from build123d import *

# Parameters (mm, degrees)
SKETCH1_R           = 2.45
SKETCH1_W           = 10
SKETCH1_H           = 3.175
SKETCH1_W_2         = 12
SKETCH1_H_2         = 2
BOSS_EXTRUDE1_DEPTH = 3.175


with BuildPart() as part:
    # Sketch1 → Boss-Extrude1 (new body)
    with BuildSketch(Plane(origin=(0, 0, 0), x_dir=(1, 0, 0), z_dir=(0, 1, 0))):
        Polygon((0, 0), (100, 0), (100, 10), (103.175, 10), (103.175, 20), (100, 20), (100, 80), (103.175, 80), (103.175, 90), (100, 90), (100, 100), (0, 100), (0, 90), (-3.175, 90), (-3.175, 80), (0, 80), (0, 20), (-3.175, 20), (-3.175, 10), (0, 10), align=None)
        with Locations((12.5, 70)):
            Circle(SKETCH1_R, mode=Mode.SUBTRACT)
        with Locations((37.5, 70)):
            Circle(SKETCH1_R, mode=Mode.SUBTRACT)
        with Locations((62.5, 70)):
            Circle(SKETCH1_R, mode=Mode.SUBTRACT)
        with Locations((87.5, 70)):
            Circle(SKETCH1_R, mode=Mode.SUBTRACT)
        with Locations((15, 95.2375)):
            Rectangle(SKETCH1_W, SKETCH1_H, mode=Mode.SUBTRACT)
        with Locations((85, 95.2375)):
            Rectangle(SKETCH1_W, SKETCH1_H, mode=Mode.SUBTRACT)
        with Locations((85, 4.7625)):
            Rectangle(SKETCH1_W, SKETCH1_H, mode=Mode.SUBTRACT)
        with Locations((15, 4.7625)):
            Rectangle(SKETCH1_W, SKETCH1_H, mode=Mode.SUBTRACT)
        with Locations((37.5, 35)):
            Rectangle(SKETCH1_W_2, SKETCH1_H_2, mode=Mode.SUBTRACT)
        with Locations((12.5, 35)):
            Rectangle(SKETCH1_W_2, SKETCH1_H_2, mode=Mode.SUBTRACT)
        with Locations((12.5, 26)):
            Rectangle(SKETCH1_W_2, SKETCH1_H_2, mode=Mode.SUBTRACT)
        with Locations((37.5, 26)):
            Rectangle(SKETCH1_W_2, SKETCH1_H_2, mode=Mode.SUBTRACT)
        with Locations((62.5, 35)):
            Rectangle(SKETCH1_W_2, SKETCH1_H_2, mode=Mode.SUBTRACT)
        with Locations((62.5, 26)):
            Rectangle(SKETCH1_W_2, SKETCH1_H_2, mode=Mode.SUBTRACT)
        with Locations((87.5, 35)):
            Rectangle(SKETCH1_W_2, SKETCH1_H_2, mode=Mode.SUBTRACT)
        with Locations((87.5, 26)):
            Rectangle(SKETCH1_W_2, SKETCH1_H_2, mode=Mode.SUBTRACT)
    extrude(amount=BOSS_EXTRUDE1_DEPTH)


solid = part.part
Here's how the part is built. I have some questions about the finished solid (model axes, mm). A direction names the side the tool comes from. Coordinates: 2 decimals unless noted, no trailing zeros. Write each loop counter-clockwise with the first axis right and the second up, starting at its lowest first coordinate (ties: lowest second). Pieces come first, ordered by that corner, then holes.
Item 1: On a 3-axis mill with a long thin cutter (end or side, diameter ignored), from which of +Z, -Z, +X, -X, +Y, -Y can I reach the whole of each face in a straight line? I mean faces 4 (the flat face through (103.175, 2, -15)), 5 (the flat face through (87, 2, -25)), 6 (the flat face through (100, 2, -95)). Say none if no direction works.
Item 2: I want a section at B-B on x = 37.5. Write out the boundary of the cut face in (y, z) (3 decimals), and give its area (3 significant figures).
Item 3: I want a section at C-C on x = 12.5. Write out the boundary of the cut face in (y, z) (3 decimals).
Item 4: If we mould it in two halves opening along Z, with no side actions, what happens to faces 1 (the flat face through (49, 2, 0)), 2 (the flat face through (85, 2, -3.175)), 3 (the flat face through (-3.175, 2, -85))? For each: +Z half, -Z half, draft (parallel to the pull), parting line (faces both ways), or undercut.
Item 5: I want a section at A-A on z = -70. Write out the boundary of the cut face in (x, y) (3 decimals).
Item 6: I want a section at D-D on y = 1.6. Count the separate pieces of the cut face and the enclosed holes in it, and give its area (3 significant figures).
Item 7: Will these pins go through, and if not, where does the flat tip stop? pin 1 (1.6 mm diameter, centred on y = 1.5, z = -35, fed in from -X); pin 2 (1 mm diameter, centred on y = 1.5, z = -94.5, fed in from +X).
Item 8: If I drill on line 1 (Z direction, x = 62.5, y = 1.9); line 2 (Z direction, x = 67.5, y = 2.2); line 3 (X direction, y = 2.4, z = -70), over which ranges is the centre line in solid material (lowest first)?
Findings below:
1. face 4: +Z, -Z, +X, +Y, -Y
1. face 5: +Y, -Y
1. face 6: -Z, +X, +Y, -Y
2. outline: (0, -100) - (3.175, -100) - (3.175, -72.45) - (0, -72.45) - close; (0, -67.55) - (3.175, -67.55) - (3.175, -36) - (0, -36) - close; (0, -34) - (3.175, -34) - (3.175, -27) - (0, -27) - close; (0, -25) - (3.175, -25) - (3.175, 0) - (0, 0) - close
2. area: 289 mm2
3. outline: (0, -100) - (3.175, -100) - (3.175, -96.825) - (0, -96.825) - close; (0, -93.65) - (3.175, -93.65) - (3.175, -72.45) - (0, -72.45) - close; (0, -67.55) - (3.175, -67.55) - (3.175, -36) - (0, -36) - close; (0, -34) - (3.175, -34) - (3.175, -27) - (0, -27) - close; (0, -25) - (3.175, -25) - (3.175, -6.35) - (0, -6.35) - close; (0, -3.175) - (3.175, -3.175) - (3.175, 0) - (0, 0) - close
4. face 1: +Z half
4. face 2: undercut
4. face 3: draft
5. outline: (0, 0) - (10.05, 0) - (10.05, 3.175) - (0, 3.175) - close; (14.95, 0) - (35.05, 0) - (35.05, 3.175) - (14.95, 3.175) - close; (39.95, 0) - (60.05, 0) - (60.05, 3.175) - (39.95, 3.175) - close; (64.95, 0) - (85.05, 0) - (85.05, 3.175) - (64.95, 3.175) - close; (89.95, 0) - (100, 0) - (100, 3.175) - (89.95, 3.175) - close
6. separate pieces: 1
6. enclosed holes: 16
6. area: 9,730 mm2
7. pin 1: stops at x = 0
7. pin 2: stops at x = 100
8. line 1: z = -100 to -72.45, -67.55 to -36, -34 to -27, -25 to 0
8. line 2: z = -100 to -36, -34 to -27, -25 to 0
8. line 3: x = 0 to 10.05, 14.95 to 35.05, 39.95 to 60.05, 64.95 to 85.05, 89.95 to 100
